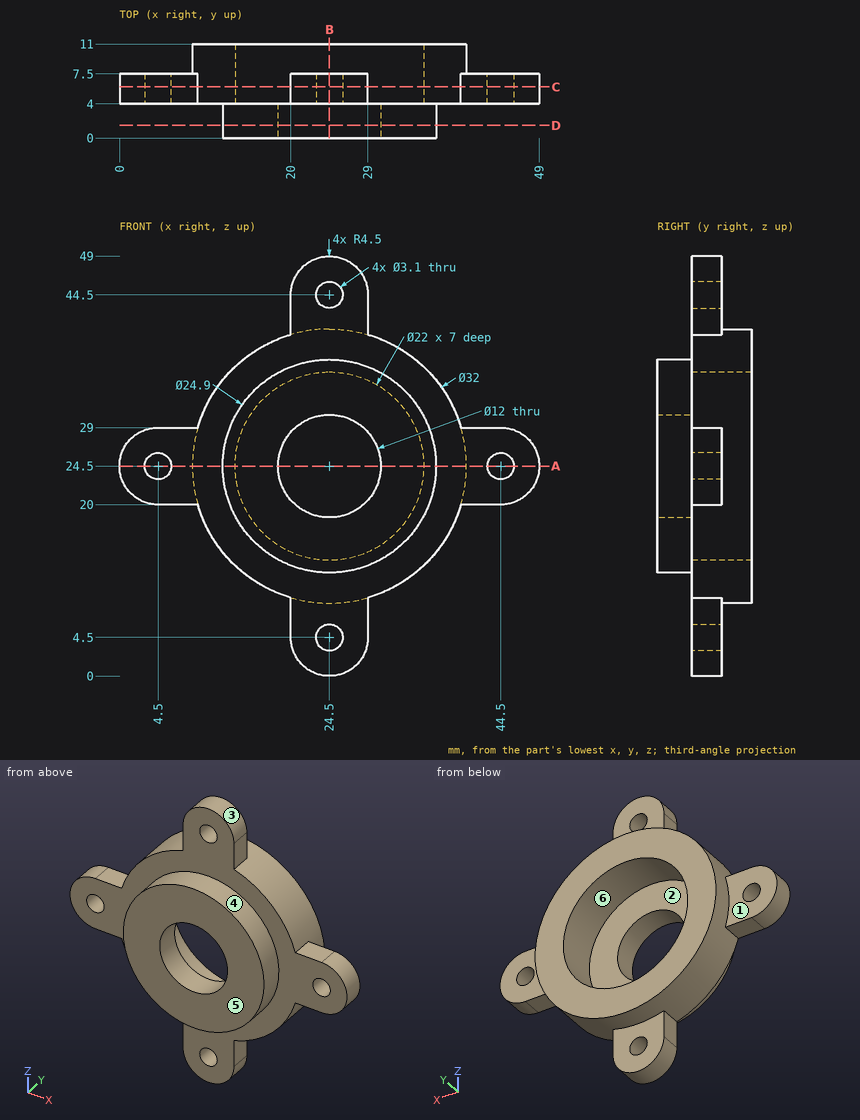
The drawing under review shows one solid part. Ordinate dimensions are in mm from its lowest x, y, z. A direction names the side the tool comes from. Round coordinates to 2 decimals unless told otherwise and drop trailing zeros. Write each loop counter-clockwise with the first axis right and the second up, starting at its lowest first coordinate (ties: lowest second). Pieces come first, ordered by that corner, then holes. Notation, with made-up numbers: (-10, 13) -> (24, 13) arc R29 ccw to (24, 47) -> close; hole circle Ø7 at (89.5, -37.75). An arc over 180 degrees is marked (long way). One line per question, with ' | ' between items. Start each with the question number.
(1) Add section B-B, the plane x = 24.5. Write out the cut boundary in (y, z), plus the area to 3 significant figures.
(2) Add section A-A, the plane z = 24.5. Write out the cut boundary in (x, y), plus the area to 3 significant figures.
(3) Mouldability with a two-part tool opening along X and no side actions: class the marked faces 1, 2 and 3 as released by +X, released by -X, zero draft, split by the parting line, or undercut.
(4) Add section D-D, the plane y = 1.5. Write out the cut boundary in (x, z), plus the area to 3 significant figures.
(5) Tool access review of the marked faces 4, 5 and 6: name each direction out of +Z, -Z, +X, -X, +Y, -Y from which nothing blocks a thin tool from reaching the whole face with its end or side.
(6) Insertion check: P1, Ø1, axis at y = 9, z = 5, coming from the +X side; P2, Ø4, axis at y = 5, z = 6, coming from the +X side; P3, Ø2.5, axis at x = 25.5, z = 4, coming from the +Y side; P4, Ø2, axis at x = 22, y = 9.5, coming from the +Z side. Each pin has a flat end and moves straight along its axis. Give the tip position at first contact, or say it passes through.
(7) For line 1 along X through (y, z) = (1.75, 24.5); line 2 along Y through (x, z) = (31.5, 12); line 3 along X through (y, z) = (6.25, 4.5), list the stretches that pass through material, from the lowest coordinate up. Write a range as from..to.
(8) Add section C-C, the plane y = 6. Write out the cut boundary in (x, z), plus the area to 3 significant figures.
Answer list:
1) outline: (0, 12.05) -> (4, 12.05) -> (4, 6.05) -> (7.5, 6.05) -> (7.5, 8.5) -> (11, 8.5) -> (11, 13.5) -> (4, 13.5) -> (4, 18.5) -> (0, 18.5) -> close; (0, 30.5) -> (4, 30.5) -> (4, 35.5) -> (11, 35.5) -> (11, 40.5) -> (7.5, 40.5) -> (7.5, 42.95) -> (4, 42.95) -> (4, 36.95) -> (0, 36.95) -> close; (4, 0) -> (7.5, 0) -> (7.5, 2.95) -> (4, 2.95) -> close; (4, 46.05) -> (7.5, 46.05) -> (7.5, 49) -> (4, 49) -> close | area: 159 mm²
2) outline: (0, 4) -> (2.95, 4) -> (2.95, 7.5) -> (0, 7.5) -> close; (6.05, 4) -> (12.05, 4) -> (12.05, 0) -> (18.5, 0) -> (18.5, 4) -> (13.5, 4) -> (13.5, 11) -> (8.5, 11) -> (8.5, 7.5) -> (6.05, 7.5) -> close; (30.5, 0) -> (36.95, 0) -> (36.95, 4) -> (42.95, 4) -> (42.95, 7.5) -> (40.5, 7.5) -> (40.5, 11) -> (35.5, 11) -> (35.5, 4) -> (30.5, 4) -> close; (46.05, 4) -> (49, 4) -> (49, 7.5) -> (46.05, 7.5) -> close | area: 159 mm²
3) face 1: zero draft | face 2: undercut | face 3: split by the parting line
4) outline: circle Ø24.9 at (24.5, 24.5); hole circle Ø12 at (24.5, 24.5) | area: 374 mm²
5) face 4: -Y | face 5: +Z, -Z, +X, -X, -Y | face 6: +Y
6) P1: through | P2: x = 29 | P3: y = 7.5 | P4: z = 40.43
7) line 1: 12.05..18.5, 30.5..36.95 | line 2: 4..11 | line 3: 20..22.95, 26.05..29
8) outline: (4.5, 20) -> (9.15, 20) arc R16 ccw to (20, 9.15) -> (20, 4.5) arc R4.5 ccw to (29, 4.5) -> (29, 9.15) arc R16 ccw to (39.85, 20) -> (44.5, 20) arc R4.5 ccw to (44.5, 29) -> (39.85, 29) arc R16 ccw to (29, 39.85) -> (29, 44.5) arc R4.5 ccw to (20, 44.5) -> (20, 39.85) arc R16 ccw to (9.15, 29) -> (4.5, 29) arc R4.5 ccw to start; hole circle Ø3.1 at (4.5, 24.5); hole circle Ø22 at (24.5, 24.5); hole circle Ø3.1 at (24.5, 4.5); hole circle Ø3.1 at (24.5, 44.5); hole circle Ø3.1 at (44.5, 24.5) | area: 673 mm²
